Geometry: see drawing. Coordinates: mm, zero at the bounding-box minimum. A direction names the side the tool comes from. Round coordinates to 2 decimals unless told otherwise and drop trailing zeros. Order: outer loops, then holes, each group sorted by start corner. A loop starts at its lowest first (then second) coordinate and runs counter-clockwise, first axis right, second up. Notation, with made-up numbers: (76, 86) -> (102, 86) arc R11 cw to (102, 101) -> close; hole circle Ø10 at (59, 44.5). An arc over 180 degrees is marked (long way). Answer as CSV lines item,"result". Start each with the question number.
(1) Set-up query: the marked faces 1, 2, 3 and 4. Return all of +Z, -Z, +X, -X, +Y, -Y with unobstructed straight access to the full face (end or side cutting, diameter ignored); none if empty.
(2) Section query B-B (x = 7.5). Output: boundary loops of the cut face in (y, z), plus the area to 3 significant figures.
(3) Pull-direction query (X, two-part tool) for the marked faces 5, 6 and 7; classes: +X half, -X half, draft (parallel to the pull), parting line (faces both ways), or undercut.
(4) Section query D-D (x = 4.75). Output: boundary loops of the cut face in (y, z).
(5) Line query: line 1 along Z through (x, y) = (3.75, 2.9); line 2 along X through (y, z) = (0.7, 6.75); line 3 along X through (y, z) = (0.35, 9.5). Output: solid intervals per line, ascending. Write a range as from..to.
(6) Section query A-A (z = 8.5). Output: boundary loops of the cut face in (x, y), plus the area to 3 significant figures.
(7) Section query C-C (y = 1.25). Output: boundary loops of the cut face in (x, z), plus the area to 3 significant figures.
(8) Contact query for flat-ended pins moving along their axis: P1, Ø0.9, axis at y = 1.5, z = 1, coming from the -X side; P2, Ø0.5, axis at x = 9.5, y = 1.5, coming from the -Z side. Output: stop coordinate, or through.
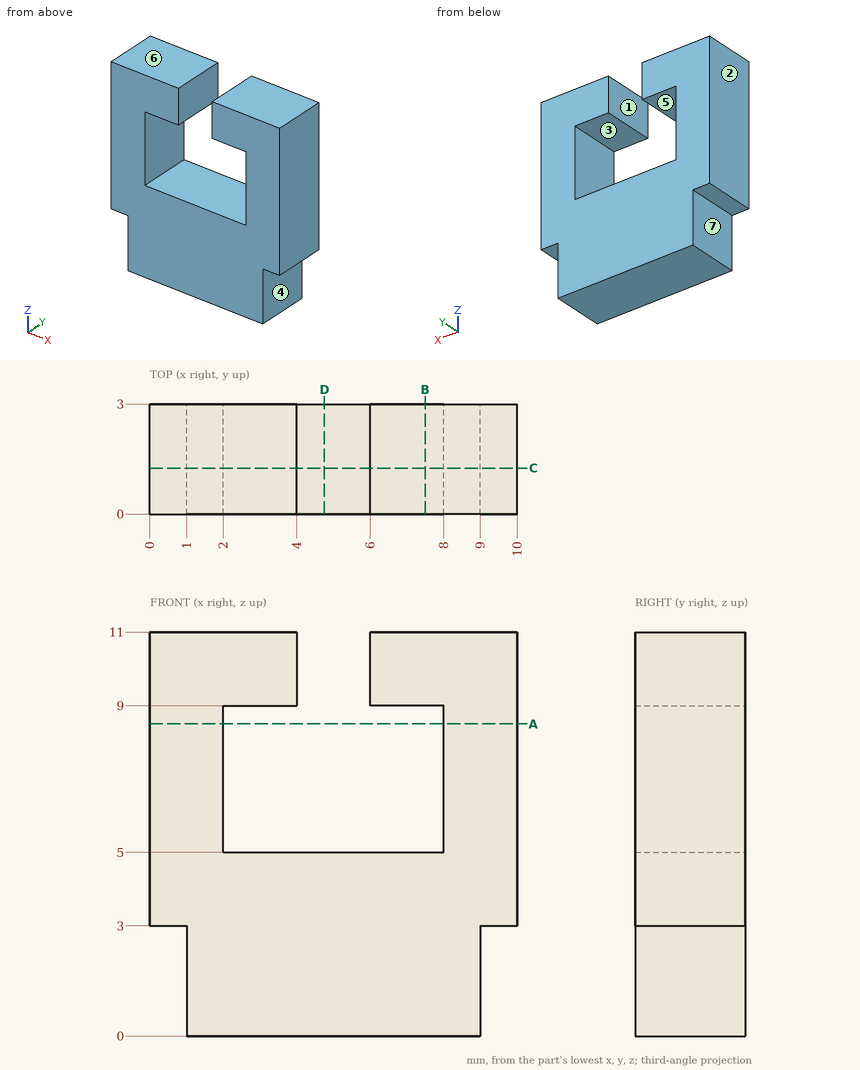
Answer block:
1,face 1,"+Z, +Y, -Y"
1,face 2,"+Z, -Z, -X, +Y, -Y"
1,face 3,"+Y, -Y"
1,face 4,"-Z, +X, +Y, -Y"
2,outline,"(0, 0) -> (3, 0) -> (3, 5) -> (0, 5) -> close; (0, 9) -> (3, 9) -> (3, 11) -> (0, 11) -> close"
2,area,"21.0 mm2"
3,face 5,"undercut"
3,face 6,"draft"
3,face 7,"-X half"
4,outline,"(0, 0) -> (3, 0) -> (3, 5) -> (0, 5) -> close"
5,line 1,"0..5, 9..11"
5,line 2,"0..2, 8..10"
5,line 3,"0..4, 6..10"
6,outline,"(0, 0) -> (2, 0) -> (2, 3) -> (0, 3) -> close; (8, 0) -> (10, 0) -> (10, 3) -> (8, 3) -> close"
6,area,"12.0 mm2"
7,outline,"(0, 3) -> (1, 3) -> (1, 0) -> (9, 0) -> (9, 3) -> (10, 3) -> (10, 11) -> (6, 11) -> (6, 9) -> (8, 9) -> (8, 5) -> (2, 5) -> (2, 9) -> (4, 9) -> (4, 11) -> (0, 11) -> close"
7,area,"76.0 mm2"
8,P1,"x = 1"
8,P2,"z = 3"
